Autodesk Inventor part; units mm, degrees
ref_plane "YZ Plane" through (0, 0, 0) normal (1, 0, 0) x (0, 1, 0)
ref_plane "XZ Plane" through (0, 0, 0) normal (0, 1, 0) x (-1, 0, 0)
ref_plane "XY Plane" through (0, 0, 0) normal (0, 0, 1) x (1, 0, 0)
sketch "Sketch1" plane through (0, 0, 0) normal (0, 0, 1) x (1, 0, 0)
  line L0 (0, 0) -> (114, 0)
  line L1 (114, 0) -> (114, 114)
  line L2 (114, 114) -> (0, 114)
  line L3 (0, 114) -> (0, 0)
  dimension "d0" = 114
  dimension "d1" = 114
extrude "Extrusion1" add sketch "Sketch1" along normal blind 200
fillet "Fillet1" radius 10 1 edges at (0, 114, 100)
fillet "Fillet2" radius 10 3 edges at (114, 114, 100) (114, 0, 100) (0, 0, 100)
sketch "Sketch3" plane through (0, 0, 200) normal (0, 0, 1) x (1, 0, 0)
  circle A0 centre (11.038, 11.038) radius 4.5
  line L0 (10, 0) -> (104, 0)
  line L1 (0, 104) -> (0, 10)
  circle A1 centre (11.038, 102.962) radius 4.5
  circle A2 centre (102.962, 102.962) radius 4.5
  circle A3 centre (102.962, 11.038) radius 4.5
  line L2 (104, 114) -> (10, 114)
  line L3 (114, 10) -> (114, 104)
  point P0 (0, 0)
  dimension "d11" = 9
  dimension "d12" = 11.038
  dimension "d13" = 11.038
  dimension "d14" = 9
  dimension "d15" = 9
  dimension "d16" = 9
  dimension "d17" = 11.038
  dimension "d18" = 11.038
  dimension "d19" = 11.038
  dimension "d20" = 11.038
  dimension "d21" = 11.038
  dimension "d22" = 11.038
extrude "Extrusion3" cut sketch "Sketch3" against normal blind 500
sketch "Sketch6" plane through (0, 0, 200) normal (0, 0, 1) x (1, 0, 0)
  arc A0 (0, 10) -> (10, 0) centre (10, 10) ccw
  line L0 (0, 10) -> (0, 24.5)
  line L1 (0, 104) -> (0, 10)
  line L2 (0, 24.5) -> (10.13, 24.5)
  line L3 (10, 0) -> (24.5, 0)
  line L4 (10, 0) -> (104, 0)
  line L5 (24.5, 0) -> (24.5, 10.13)
  arc A1 (10.13, 24.5) -> (24.5, 10.13) centre (37.2744, 37.2744) ccw
  arc A2 (10, 114) -> (0, 104) centre (10, 104) ccw
  line L6 (10, 114) -> (24.5, 114)
  line L7 (104, 114) -> (10, 114)
  line L8 (24.5, 114) -> (24.5, 103.87)
  line L9 (0, 104) -> (0, 89.5)
  line L10 (0, 89.5) -> (10.13, 89.5)
  arc A3 (24.5, 103.87) -> (10.13, 89.5) centre (37.2744, 76.7256) ccw
  line L11 (104, 114) -> (89.5, 114)
  line L12 (89.5, 114) -> (89.5, 103.87)
  line L13 (114, 10) -> (114, 104)
  line L14 (114, 104) -> (114, 89.5)
  line L15 (114, 89.5) -> (114, 99.63)
  arc A4 (103.87, 89.5) -> (89.5, 103.87) centre (76.7256, 76.7256) ccw
  line L16 (103.87, 89.5) -> (114, 89.5)
  line L17 (114, 10) -> (114, 24.5)
  line L18 (114, 24.5) -> (103.87, 24.5)
  line L19 (104, 0) -> (89.5, 0)
  line L20 (89.5, 0) -> (89.5, 10.13)
  arc A5 (89.5, 10.13) -> (103.87, 24.5) centre (76.7256, 37.2744) ccw
  point P0 (0, 0)
  dimension "d30" = 14.5
  dimension "d31" = 10.13
  dimension "d32" = 14.5
  dimension "d33" = 10.13
  dimension "d34" = 30
  dimension "d35" = 14.5
  dimension "d36" = 10.13
  dimension "d37" = 14.5
  dimension "d38" = 10.13
  dimension "d39" = 30
  dimension "d40" = 14.5
  dimension "d41" = 10.13
  dimension "d42" = 14.5
  dimension "d44" = 30
  dimension "d45" = 10.13
  dimension "d46" = 14.5
  dimension "d47" = 10.13
  dimension "d48" = 14.5
  dimension "d49" = 10.13
  dimension "d50" = 30
extrude "Extrusion5" cut sketch "Sketch6" against normal blind 146 and the other way blind 73 contours L1 L10 A3 L8 L7 L12 A4 L16 L13 L18 A5 L20 L4 L5 A1 L2
sketch "Sketch7" plane through (0, 0, 0) normal (0, 0, -1) x (-1, 0, 0)
  line L0 (0, 104) -> (0, 10)
  line L1 (-10, 0) -> (-104, 0)
  circle A0 centre (-57, 57) radius 55
  point P0 (0, 0)
  dimension "d58" = 110
extrude "Extrusion6" cut sketch "Sketch7" against normal blind 3
sketch "Sketch9" plane through (57, 57, 3) normal (0, 0, -1) x (-1, 0, 0)
  circle A0 centre (0, 0) radius 12
  line L0 (47, -57) -> (-47, -57)
  line L1 (57, 47) -> (57, -47)
  point P0 (57, -57)
  point P1 (0, -57)
  dimension "d66" = 24
  dimension "d68" = 57
  dimension "d69" = 57
extrude "Extrusion8" cut sketch "Sketch9" against normal blind 48
sketch "Sketch10" plane through (57, 57, 3) normal (0, 0, -1) x (-1, 0, 0)
  circle A0 centre (0, 0) radius 12
  line L0 (12, 0) -> (15, 0)
  line L1 (15, 4) -> (15, -4)
  line L2 (15, 4) -> (11.3137, 4)
  line L3 (15, -4) -> (11.3137, -4)
  point P0 (57, -57)
  dimension "d72" = 15
  dimension "d73" = 8
  dimension "d74" = 4
  dimension "d75" = 57
  dimension "d76" = 42
extrude "Extrusion9" cut sketch "Sketch10" against normal blind 48 contours L0 L1 L3 A0 | A0 L2 L1 L0
equation "\"d13\" = d12"
equation "\"d17\" = d12"
equation "\"d18\" = d13"
equation "\"d19\" = d18"
equation "\"d20\" = d18"
equation "\"d21\" = d19"
equation "\"d22\" = d21"
equation "\"d33\" = d31"
properties part number "BackPlate"
The model under review builds one solid part; all positions refer to its coordinate system, in mm. A direction names the side the tool comes from. Round coordinates to 2 decimals unless told otherwise and drop trailing zeros. Write each loop counter-clockwise with the first axis right and the second up, starting at its lowest first coordinate (ties: lowest second). Pieces come first, ordered by that corner, then holes. Notation, with made-up numbers: (86, 64.25) - (113, 64.25) arc R9 ccw to (113, 68.25) - close; hole circle Ø4 at (47.25, 43). An arc over 180 degrees is marked (long way). Use one line per item in the form item = value.
Q1. Consider section B-B (z = 187). State the section outline as (x, y) points, and give its area (3 significant figures).
Answer key:
outline = (0, 10) arc R10 ccw to (10, 0) - (24.5, 0) - (24.5, 10.13) arc R30 cw to (10.13, 24.5) - (0, 24.5) - close; (0, 89.5) - (10.13, 89.5) arc R30 cw to (24.5, 103.87) - (24.5, 114) - (10, 114) arc R10 ccw to (0, 104) - close; (89.5, 0) - (104, 0) arc R10 ccw to (114, 10) - (114, 24.5) - (103.87, 24.5) arc R30 cw to (89.5, 10.13) - close; (89.5, 103.87) arc R30 cw to (103.87, 89.5) - (114, 89.5) - (114, 104) arc R10 ccw to (104, 114) - (89.5, 114) - close; hole circle Ø9 at (11.04, 11.04); hole circle Ø9 at (11.04, 102.96); hole circle Ø9 at (102.96, 11.04); hole circle Ø9 at (102.96, 102.96)
area = 1,550 mm2
Q2. Tool access review of faces 1 (the cylindrical face through (69, 57, 27)), 2 (the flat face through (7, 7, 200)), 3 (the cylindrical face through (16.16, 98.04, 128.02)), 4 (the flat face through (5, 24.5, 128)), 5 (the flat face through (89.5, 5, 128)): name each direction out of +Z, -Z, +X, -X, +Y, -Y from which nothing blocks a thin tool from reaching the whole face with its end or side.
Answer key:
face_1 = -Z
face_2 = +Z, +X, -X, +Y, -Y
face_3 = +Z
face_4 = +Z, +X, -X
face_5 = +Z, +Y, -Y
Q3. Insertion check: pin 1 Ø5 at (x, z) = (108, 146) entering from +Y; pin 2 Ø12 at (x, z) = (83, 147.5) entering from -Y; pin 3 Ø5 at (x, z) = (4.5, 140) entering from +Y; pin 4 Ø3 at (x, z) = (5.5, 121.5) entering from -Y. Each pin has a flat end and moves straight along its axis. Give the tip position at first contact, or say it passes through.
Answer key:
pin_1 = 113.89
pin_2 = through
pin_3 = 113.54
pin_4 = 0.46
Q4. Draft analysis for pull direction Y (two halves, no side actions). For faces 6 (the cylindrical face through (3.01, 111.15, 101.4)), 7 (the flat face through (107, 107, 200)), 8 (the cylindrical face through (98.04, 97.84, 128.02)), state which applies: +Y half, -Y half, draft (parallel to the pull), parting line (faces both ways), or undercut.
Answer key:
face_6 = +Y half
face_7 = draft
face_8 = undercut
Q5. Consider section C-C (x = 73). State the section outline as (y, z) points.
Answer key:
outline = (0, 0) - (4.38, 0) - (4.38, 3) - (109.62, 3) - (109.62, 0) - (114, 0) - (114, 54) - (0, 54) - close
Q6. Consider section D-D (z = 18). State the section outline as (x, y) points.
Answer key:
outline = (0, 10) arc R10 ccw to (10, 0) - (104, 0) arc R10 ccw to (114, 10) - (114, 104) arc R10 ccw to (104, 114) - (10, 114) arc R10 ccw to (0, 104) - close; hole circle Ø9 at (11.04, 11.04); hole circle Ø9 at (11.04, 102.96); hole (42, 53) - (45.69, 53) arc R12 ccw (long way) to (45.69, 61) - (42, 61) - close; hole circle Ø9 at (102.96, 11.04); hole circle Ø9 at (102.96, 102.96)
Q7. For line 1 (Y direction, x = 57, z = 14); line 2 (Y direction, x = 15, z = 175); line 3 (Z direction, x = 30, y = 44), list the stretches that pass through material, from the lowest coordinate up. Write a range as [from, to].
Answer key:
line_1 = [0, 45], [69, 114]
line_2 = [0, 8.9], [13.17, 17.18], [96.82, 100.83], [105.1, 114]
line_3 = [3, 54]
Q8. Consider section A-A (y = 57). State the section outline as (x, z) points, and give its area (3 significant figures).
Answer key:
outline = (0, 0) - (2, 0) - (2, 3) - (42, 3) - (42, 51) - (69, 51) - (69, 3) - (112, 3) - (112, 0) - (114, 0) - (114, 54) - (0, 54) - close
area = 4,530 mm2
